```python
from build123d import *

# Parameters (mm, degrees)
SKETCH_1_W          = 60
SKETCH_1_H          = 27
EXTRUDE_1_DEPTH     = 3
SKETCH_2_W          = 150
SKETCH_2_H          = 6
EXTRUDE_2_DEPTH     = 3
EXTRUDE_3_DEPTH     = 3
SKETCH_4_R          = 1.7
CUT_EXTRUDE_1_DEPTH = 98.67420335
EXTRUDE_4_DEPTH     = 3
SKETCH_6_R          = 2.7
CUT_EXTRUDE_2_DEPTH = 98.67420335


with BuildPart() as part:
    # 草圖1 → 填料-伸長1 (new body)
    with BuildSketch(Plane.XY):
        Rectangle(SKETCH_1_W, SKETCH_1_H)
    extrude(amount=EXTRUDE_1_DEPTH)

    # 草圖2 → 填料-伸長2 (add)
    with BuildSketch(Plane.XY.offset(3)):
        with Locations((0, -10.5)):
            Rectangle(SKETCH_2_W, SKETCH_2_H)
    extrude(amount=-EXTRUDE_2_DEPTH)

    # 草圖3 → 填料-伸長3 (add)
    with BuildSketch(Plane.XY.offset(3)):
        Polygon((65, -62.5), (75, -62.5), (75, -7.5), (-75, -7.5), (-75, -62.5), (-65, -62.5), (-65, -13.5), (65, -13.5), align=None)
    extrude(amount=-EXTRUDE_3_DEPTH)

    # 草圖4 → 除料-伸長1 (cut, through all)
    with BuildSketch(Plane.XY.offset(3)):
        with Locations((-72, -10.5)):
            Circle(SKETCH_4_R)
        with Locations(Location((-72, -59.5, 0), (0, 0, 180))):
            Circle(SKETCH_4_R)
        with Locations((72, -59.5)):
            Circle(SKETCH_4_R)
        with Locations(Location((72, -10.5, 0), (0, 0, 180))):
            Circle(SKETCH_4_R)
    extrude(amount=-CUT_EXTRUDE_1_DEPTH, mode=Mode.SUBTRACT)

    # 草圖5 → 填料-伸長4 (add)
    with BuildSketch(Plane.XY.offset(3)):
        Polygon((-63.853075311, -39.638463841), (-28.853075311, -15.138463841), (-26.512412681, -13.5), (-33.487587319, -13.5), (-65, -35.558688877), (-65, -38), (-65, -40.441311123), align=None)
        Polygon((26.512412681, -13.5), (33.487587319, -13.5), (65, -35.558688877), (65, -38), (65, -40.441311123), (63.853075311, -39.638463841), (28.853075311, -15.138463841), align=None)
    extrude(amount=-EXTRUDE_4_DEPTH)

    # 草圖6 → 除料-伸長2 (cut, through all)
    with BuildSketch(Plane.XY.offset(3)):
        with Locations((-18, 3.5)):
            Circle(SKETCH_6_R)
        with Locations(Location((18, 3.5, 0), (0, 0, 180))):
            Circle(SKETCH_6_R)
    extrude(amount=-CUT_EXTRUDE_2_DEPTH, mode=Mode.SUBTRACT)


solid = part.part
```
Check sheet for the modelled part. Datum: model origin and axes. Units: mm. A direction names the side the tool comes from. Coordinates: 2 decimals unless noted, no trailing zeros. Write each loop counter-clockwise with the first axis right and the second up, starting at its lowest first coordinate (ties: lowest second). Pieces come first, ordered by that corner, then holes. Notation, with made-up numbers: (-20.75, 4) -> (-8.75, 4) arc R20 ccw to (-8.75, 15) -> close; hole circle Ø1 at (47, 22.25). An arc over 180 degrees is marked (long way). Use a Markdown table: item, result.
1. Sectioned sample at A-A (x = 72). Enter the section's corners in (y, z).
Reported:
| item | result |
|---|---|
| outline | (-62.5, 0) -> (-61.2, 0) -> (-61.2, 3) -> (-62.5, 3) -> close; (-57.8, 0) -> (-12.2, 0) -> (-12.2, 3) -> (-57.8, 3) -> close; (-8.8, 0) -> (-7.5, 0) -> (-7.5, 3) -> (-8.8, 3) -> close |
2. Sectioned sample at D-D (x = -18). Enter the section's corners in (y, z).
Reported:
| item | result |
|---|---|
| outline | (-13.5, 0) -> (0.8, 0) -> (0.8, 3) -> (-13.5, 3) -> close; (6.2, 0) -> (13.5, 0) -> (13.5, 3) -> (6.2, 3) -> close |
3. Tool access check on faces 4 (the flat face through (-70, -62.5, 2)), 5 (the flat face through (-49, -13.5, 2)), 6 (the flat face through (52, -7.5, 2)), 7 (the flat face through (0, -10, 3)), 8 (the flat face through (-65, -52, 2)). Record the directions out of +Z, -Z, +X, -X, +Y, -Y that give a thin tool (end or side, any length) a straight path to the whole face; none if there is none.
Reported:
| item | result |
|---|---|
| face 4 | +Z, -Z, +X, -X, -Y |
| face 5 | +Z, -Z |
| face 6 | +Z, -Z, +X, +Y |
| face 7 | +Z, +X, -X, +Y, -Y |
| face 8 | +Z, -Z, -Y |
4. Sectioned sample at C-C (z = 0.6). Give the number of separate pieces and of enclosed holes in the cut face, plus the area to 3 significant figures.
Reported:
| item | result |
|---|---|
| separate pieces | 1 |
| enclosed holes | 8 |
| area | 3,400 mm2 |
5. Sectioned sample at B-B (y = 3.5). Enter the section's corners in (x, z).
Reported:
| item | result |
|---|---|
| outline | (-30, 0) -> (-20.7, 0) -> (-20.7, 3) -> (-30, 3) -> close; (-15.3, 0) -> (15.3, 0) -> (15.3, 3) -> (-15.3, 3) -> close; (20.7, 0) -> (30, 0) -> (30, 3) -> (20.7, 3) -> close |
6. Release check for a two-part mould opening along X. For faces 1 (the cylindrical face through (-70.3, -59.57, 1.52)), 2 (the flat face through (-30, 3, 1)), 3 (the flat face through (70, -62.5, 2)) record: pulls with the +X half, pulls with the -X half, needs draft (parallel to the pull), parting line crosses it, or undercut.
Reported:
| item | result |
|---|---|
| face 1 | undercut |
| face 2 | pulls with the -X half |
| face 3 | needs draft |
7. Go/stop test with flat-tipped pins: pin 1 Ø0.9 at (x, z) = (-61.5, 1) entering from +Y; pin 2 Ø0.9 at (y, z) = (-1, 1.5) entering from +X; pin 3 Ø5.5 at (x, y) = (72, -59.5) entering from -Z; pin 4 Ø1.5 at (x, z) = (-28, 0.5) entering from -Y. Record where each tip stops, or that it passes through.
Reported:
| item | result |
|---|---|
| pin 1 | stops at y = -7.5 |
| pin 2 | stops at x = 30 |
| pin 3 | stops at z = 0 |
| pin 4 | stops at y = -15.07 |
8. Scan lines: line 1 along Y through (x, z) = (72, 0.95); line 2 along Y through (x, z) = (-18, 1.5); line 3 along X through (y, z) = (-9.5, 2.3). Record each from-to range of solid material in increasing order.
Reported:
| item | result |
|---|---|
| line 1 | y = -62.5 to -61.2, -57.8 to -12.2, -8.8 to -7.5 |
| line 2 | y = -13.5 to 0.8, 6.2 to 13.5 |
| line 3 | x = -75 to -73.37, -70.63 to 70.63, 73.37 to 75 |
